Here's how the part is built. I have some questions about the finished solid (model axes, mm). A direction names the side the tool comes from. Round coordinates to 2 decimals unless told otherwise and drop trailing zeros. Write each loop counter-clockwise with the first axis right and the second up, starting at its lowest first coordinate (ties: lowest second). Pieces come first, ordered by that corner, then holes. Notation, with made-up numbers: (-32, -4) -> (26, -4) arc R32 cw to (26, 22) -> close; hole circle Ø6 at (70.25, 4.25). An arc over 180 degrees is marked (long way). Put each result on its own line as item: value. Start each with the question number.
1) We'd pull the mould along X, two halves only. Please class faces 4 (the flat face through (50, 21, 0)), 5 (the flat face through (-3.9, 3.8, 6)), 6 (the flat face through (-44, 38, 3.4)): released by +X, released by -X, zero draft, split by the parting line, or undercut.
2) I want a section at C-C, the plane z = 5. List the corners of the cut face in (x, y) for me.
3) I want a section at A-A, the plane z = 0. Give the number of separate pieces and of enclosed holes in the cut face, then the cut area to 3 significant figures.
4) If I drill on line 1 along X through (y, z) = (41.15, 0); line 2 along Z through (x, y) = (44, 17.5); line 3 along X through (y, z) = (14.5, 2.25), over which ranges is the centre line in solid material (lowest first)? Write a range as [from, to].
5) Will this pin go through, and if not, where does the flat tip stop? P1, Ø3, axis at x = -44, z = 0, coming from the -Y side.
6) I want a section at B-B, the plane x = 44. List the corners of the cut face in (y, z) for me.
7) I want a section at D-D, the plane x = -1.5. List the corners of the cut face in (y, z) for me, then the cut area to 3 significant figures.
8) Which directions (+Z, -Z, +X, -X, +Y, -Y) give clear straight access to the entire face, cutting with the end or side of a thin tool? Please do faces 1 (the flat face through (-44, 38, -3.4)), 2 (the cylindrical face through (42.58, 18.09, 0.74)), 3 (the flat face through (-1, 4, 0)).
from build123d import *

# Parameters (mm, degrees)
SKETCH2_W         = 100
SKETCH2_H         = 12
SKETCH2_R         = 1.6
BODY_DEPTH        = 4
SKETCH4_W         = 10
SKETCH4_H         = 12
SKETCH4_R         = 1.6
WINGS_DEPTH       = 38.1
SKETCH6_W         = 6.8
SKETCH6_H         = 2.8
CAPTIVE_NUT_DEPTH = 8.5
CIRPATTERN1_COUNT = 2


with BuildPart() as part:
    # Sketch2 → body (new body)
    with BuildSketch(Plane(origin=(0, 0, 0), x_dir=(1, 0, 0), z_dir=(0, 1, 0))):
        Rectangle(SKETCH2_W, SKETCH2_H)
        with Locations(Location((-44, 0, 0), (0, 0, 270))):
            Circle(SKETCH2_R, mode=Mode.SUBTRACT)
        with Locations(Location((44, 0, 0), (0, 0, 270))):
            Circle(SKETCH2_R, mode=Mode.SUBTRACT)
    extrude(amount=BODY_DEPTH)

    # Sketch4 → wings (add)
    # profile 1 of 2: a face of its own
    with BuildSketch(Plane(origin=(0, 4, 0), x_dir=(1, 0, 0), z_dir=(0, 1, 0))):
        with Locations((-45, 0)):
            Rectangle(SKETCH4_W, SKETCH4_H)
        with Locations(Location((-44, 0, 0), (0, 0, 270))):
            Circle(SKETCH4_R, mode=Mode.SUBTRACT)
    # profile 2 of 2: a face of its own
    with BuildSketch(Plane(origin=(0, 4, 0), x_dir=(1, 0, 0), z_dir=(0, 1, 0))):
        with Locations((45, 0)):
            Rectangle(SKETCH4_W, SKETCH4_H)
        with Locations(Location((44, 0, 0), (0, 0, 270))):
            Circle(SKETCH4_R, mode=Mode.SUBTRACT)
    extrude(amount=WINGS_DEPTH)

    # Sketch6 → captive-nut (cut)
    with BuildSketch(Plane.ZY.offset(-40)):
        with Locations((0, 38.1)):
            Rectangle(SKETCH6_W, SKETCH6_H)
    captive_nut = extrude(amount=-CAPTIVE_NUT_DEPTH, mode=Mode.SUBTRACT)

    # CirPattern1: captive-nut ×2 about axis
    cirpattern1_axis = Axis((0, 0, 0), (0, 1, 0))
    for i in range(1, CIRPATTERN1_COUNT):
        add(captive_nut.rotate(cirpattern1_axis, i * 360 / CIRPATTERN1_COUNT), mode=Mode.SUBTRACT)


solid = part.part
Findings:
1. face 4: released by +X
1. face 5: zero draft
1. face 6: undercut
2. outline: (-50, 0) -> (50, 0) -> (50, 42.1) -> (40, 42.1) -> (40, 4) -> (-40, 4) -> (-40, 42.1) -> (-50, 42.1) -> close
3. separate pieces: 5
3. enclosed holes: 0
3. area: 863 mm2
4. line 1: x = [-50, -45.6], [-42.4, -40], [40, 42.4], [45.6, 50]
4. line 2: z = [-6, -1.6], [1.6, 6]
4. line 3: x = [-50, -40], [40, 50]
5. P1: passes through
6. outline: (0, -6) -> (42.1, -6) -> (42.1, -1.6) -> (39.5, -1.6) -> (39.5, -3.4) -> (36.7, -3.4) -> (36.7, -1.6) -> (0, -1.6) -> close; (0, 1.6) -> (36.7, 1.6) -> (36.7, 3.4) -> (39.5, 3.4) -> (39.5, 1.6) -> (42.1, 1.6) -> (42.1, 6) -> (0, 6) -> close
7. outline: (0, -6) -> (4, -6) -> (4, 6) -> (0, 6) -> close
7. area: 48.0 mm2
8. face 1: none
8. face 2: +Y, -Y
8. face 3: +Z, -Z, +Y
